```python
from build123d import *

# Parameters (mm, degrees)
SZKIC1_W                    = 20
SZKIC1_H                    = 27
DODANIE_WYCI_GNI_CIE1_DEPTH = 12
ZAOKR_GLENIE2_R             = 6
SKETCH3_W                   = 6.414141748
SKETCH3_H                   = 0.7
F_3_0MM_DOWEL_HOLE2_D       = 3
F_3_0MM_DOWEL_HOLE2_DEPTH   = 2.5
F_3_0MM_DOWEL_HOLE2_TIP     = 0.901290929
F_3_0MM_DOWEL_HOLE3_D       = 3.2
F_6_0MM_DOWEL_HOLE1_D       = 7
F_6_0MM_DOWEL_HOLE1_DEPTH   = 16.6
F_3_0MM_DOWEL_HOLE4_D       = 3
F_3_0MM_DOWEL_HOLE4_DEPTH   = 3
F_3_0MM_DOWEL_HOLE4_TIP     = 0.901290929
F_5_0MM_DOWEL_HOLE1_D       = 5
F_5_0MM_DOWEL_HOLE1_DEPTH   = 2.4
F_10_0MM_DOWEL_HOLE3_D      = 10
F_10_0MM_DOWEL_HOLE3_DEPTH  = 6
F_10_0MM_DOWEL_HOLE3_TIP    = 3.004303095


with BuildPart() as part:
    # Szkic1 → Dodanie-wyciągnięcie1 (new body)
    with BuildSketch(Plane.XY):
        with Locations((10, 13.5)):
            Rectangle(SZKIC1_W, SZKIC1_H)
    extrude(amount=DODANIE_WYCI_GNI_CIE1_DEPTH)

    # Zaokrąglenie2
    zaokr_glenie2_edges = [part.edges().sort_by_distance(p)[0] for p in [
        (20, 13.5, 0),
        (20, 13.5, 12),
        (0, 13.5, 0),
        (0, 13.5, 12),
    ]]
    fillet(zaokr_glenie2_edges, radius=ZAOKR_GLENIE2_R - 0.0001)  # a hair under: the kernel refuses the full size

    # Sketch3 → Cut-Revolve1 (revolve, cut)
    with BuildSketch(Plane.ZY.offset(-10), mode=Mode.PRIVATE) as cut_revolve1_sk:
        with Locations((-1.507070874, 22.65)):
            Rectangle(SKETCH3_W, SKETCH3_H)
        with Locations((-1.507070874, 20.95)):
            Rectangle(SKETCH3_W, SKETCH3_H)
        with Locations((-1.507070874, 19.25)):
            Rectangle(SKETCH3_W, SKETCH3_H)
        with Locations((-1.507070874, 17.55)):
            Rectangle(SKETCH3_W, SKETCH3_H)
        with Locations((-1.507070874, 15.85)):
            Rectangle(SKETCH3_W, SKETCH3_H)
        with Locations((-1.507070874, 14.15)):
            Rectangle(SKETCH3_W, SKETCH3_H)
        with Locations((-1.507070874, 12.45)):
            Rectangle(SKETCH3_W, SKETCH3_H)
        with Locations((-1.507070874, 10.75)):
            Rectangle(SKETCH3_W, SKETCH3_H)
        with Locations((-1.507070874, 9.05)):
            Rectangle(SKETCH3_W, SKETCH3_H)
        with Locations((-1.507070874, 7.35)):
            Rectangle(SKETCH3_W, SKETCH3_H)
    revolve(cut_revolve1_sk.sketch.rotate(Axis((10, 26.25563002, 6), (0, -1, 0)), 180), axis=Axis((10, 26.25563002, 6), (0, -1, 0)), mode=Mode.SUBTRACT)

    # Ø3.0mm Dowel Hole2
    with Locations(Plane(origin=(0, 0, 0), x_dir=(-1, 0, 0), z_dir=(0, 0, -1))):
        with Locations((-10, 25)):
            Hole(F_3_0MM_DOWEL_HOLE2_D / 2, depth=F_3_0MM_DOWEL_HOLE2_DEPTH)
            with Locations((0, 0, -(F_3_0MM_DOWEL_HOLE2_DEPTH + F_3_0MM_DOWEL_HOLE2_TIP / 2))):  # 118° drill point
                Cone(0, F_3_0MM_DOWEL_HOLE2_D / 2, F_3_0MM_DOWEL_HOLE2_TIP, mode=Mode.SUBTRACT)

    # Ø3.0mm Dowel Hole3 (through all)
    with Locations(Plane(origin=(17.15, 4, 0), x_dir=(-1, 0, 0), z_dir=(0, 0, -1))):
        with Locations((0, 0), (14.3, 0)):
            Hole(F_3_0MM_DOWEL_HOLE3_D / 2)

    # Ø6.0mm Dowel Hole1
    with Locations(Plane(origin=(0, 27, 0), x_dir=(1, 0, 0), z_dir=(0, 1, 0))):
        with Locations((10, -6)):
            Hole(F_6_0MM_DOWEL_HOLE1_D / 2, depth=F_6_0MM_DOWEL_HOLE1_DEPTH)

    # Ø3.0mm Dowel Hole4
    with Locations(Plane(origin=(0, 27, 0), x_dir=(1, 0, 0), z_dir=(0, 1, 0))):
        with Locations((17, -7.5), (3, -7.5)):
            Hole(F_3_0MM_DOWEL_HOLE4_D / 2, depth=F_3_0MM_DOWEL_HOLE4_DEPTH)
            with Locations((0, 0, -(F_3_0MM_DOWEL_HOLE4_DEPTH + F_3_0MM_DOWEL_HOLE4_TIP / 2))):  # 118° drill point
                Cone(0, F_3_0MM_DOWEL_HOLE4_D / 2, F_3_0MM_DOWEL_HOLE4_TIP, mode=Mode.SUBTRACT)

    # Ø5.0mm Dowel Hole1
    with Locations(Plane(origin=(0, 10.4, 0), x_dir=(1, 0, 0), z_dir=(0, 1, 0))):
        with Locations((10, -6)):
            Hole(F_5_0MM_DOWEL_HOLE1_D / 2, depth=F_5_0MM_DOWEL_HOLE1_DEPTH)

    # Ø10.0mm Dowel Hole3
    with Locations(Plane(origin=(0, 0, 0), x_dir=(-1, 0, 0), z_dir=(0, -1, 0))):
        with Locations((-10, -6)):
            Hole(F_10_0MM_DOWEL_HOLE3_D / 2, depth=F_10_0MM_DOWEL_HOLE3_DEPTH)
            with Locations((0, 0, -(F_10_0MM_DOWEL_HOLE3_DEPTH + F_10_0MM_DOWEL_HOLE3_TIP / 2))):  # 118° drill point
                Cone(0, F_10_0MM_DOWEL_HOLE3_D / 2, F_10_0MM_DOWEL_HOLE3_TIP, mode=Mode.SUBTRACT)


solid = part.part
```
Here's how the part is built. I have some questions about the finished solid (model axes, mm). A direction names the side the tool comes from. Coordinates: 2 decimals unless noted, no trailing zeros. Return JSON: item names as keys, results as strings.
1) If we section it at A-A on y = 5.25: State how many separate pieces and enclosed holes the cut face has, plus the area to 3 significant figures.
Conclusion:
{"separate pieces": "3", "enclosed holes": "1", "area": "90.1 mm²"}
2) I'm going to push flat-ended pins straight in: P1, Ø1.9, axis at x = 2.85, y = 4, coming from the +Z side; P2, Ø3.5, axis at x = 10, z = 4.5, coming from the +Y side; P3, Ø2, axis at y = 16, z = 4.5, coming from the +X side; P4, Ø3.5, axis at x = 17.15, y = 4, coming from the -Z side. Where does each tip first touch, or does it pass through?
Conclusion:
{"P1": "passes through", "P2": "stops at y = 10.4", "P3": "stops at x = 19.98", "P4": "stops at z = 0.17"}
3) If I drill on probe 1 along Z at (x, y) = (10, 9.8); probe 2 along X at (y, z) = (4.5, 9.25); probe 3 along Z at (x, y) = (10, 2.75), over which ranges is the centre line in solid material (lowest first)?
Conclusion:
{"probe 1": "z = 0 to 3.5, 8.5 to 12", "probe 2": "x = 0.96 to 1.33, 4.37 to 6.2, 13.8 to 15.63, 18.67 to 19.04", "probe 3": "z = 0 to 1, 11 to 12"}
4) On a 3-axis mill with a long thin cutter (end or side, diameter ignored), from which of +Z, -Z, +X, -X, +Y, -Y can I reach the whole of each face in a straight line? I mean faces 3 (the cylindrical face through (18.2, 25.5, 8.4)), 4 (the cylindrical face through (1.05, 3.55, 9.39)). Say none if no direction works.
Conclusion:
{"face 3": "+Y", "face 4": "+Z, -X, +Y, -Y"}
5) Thinking about a two-plate mould opening in Y: for faces 1 (the cylindrical face through (1.711, 13.307, 1.804)), 2 (the flat face through (12, 16.2, 10)), which applies, +Y half, -Y half, draft (parallel to the pull), parting line (faces both ways), or undercut?
Conclusion:
{"face 1": "draft", "face 2": "undercut"}
